Part model, mm, in its own coordinate system. Face numbers are marked on the shaded views. A direction names the side the tool comes from. Round coordinates to 2 decimals unless told otherwise and drop trailing zeros. Write each loop counter-clockwise with the first axis right and the second up, starting at its lowest first coordinate (ties: lowest second). Pieces come first, ordered by that corner, then holes. Notation, with made-up numbers: M 0.25,35.5 L 35.25,35.5 A16 ccw 35.25,55.5 Z; hole C 27,2 d6. An arc over 180 degrees is marked long. Use a Markdown table: item, result. Add a question column.
1) Wall check: probe 1 along Z at (x, y) = (-3, -46); probe 2 along Y at (x, z) = (-14.5, 28); probe 3 along Z at (x, y) = (-27, -83). Give the ranges that are in metal, low to high.
2) Slice it at B-B on x = 1. Write the cut outline in (y, z).
3) Which spindle directions (+Z, -Z, +X, -X, +Y, -Y) get a long thin tool onto all of the face, cutting with end or side? Do the marked faces 1, 2, 3 and 4. Say none if no direction does.
4) Slice it at C-C on z = 51. Write the cut outline in (x, y).
5) Slice it at D-D on y = -47. Write the cut outline in (x, z), plus the area to 3 significant figures.
6) Two-plate mould, pull along Y, no slides. Class the marked faces 5, 6, 7 and 8: released by +Y, released by -Y, zero draft, split by the parting line, or undercut.
7) Drop flat-ended pins along their axis: P1, Ø5, axis at x = 2, y = -102, coming from the +Z side; P2, Ø6, axis at x = -29.5, z = 43.5, coming from the +Y side; P3, Ø12, axis at x = -27.5, z = 90.5, coming from the -Y side. Give the stop position or say it passes through.
8) Slice it at A-A on z = 126.5. Write the cut outline in (x, y).
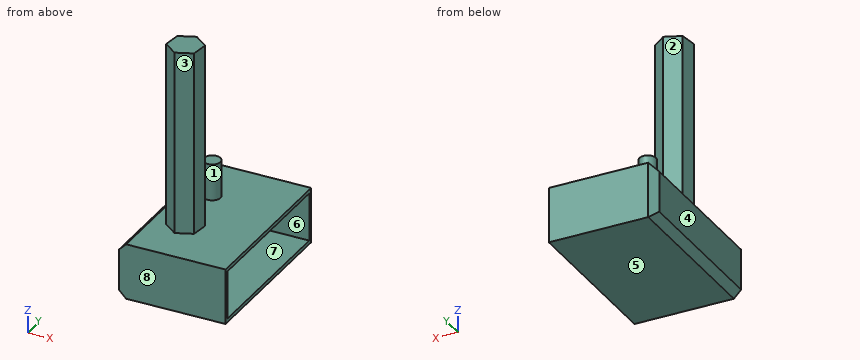
```python
from build123d import *

# Parameters (mm, degrees)
F0_W     = 74.041
F0_H     = 38.5406240821
F1_DEPTH = 115.062
F3_DEPTH = 127.762
F4_R     = 5.7167029037
F5_DEPTH = 25.4
F6_SIZE  = 5.08
F7_SIZE  = 5.08
F8_T     = -2.54


with BuildPart() as f1:
    # F0 (on Front) → F1 (new body)
    with BuildSketch(Plane.XZ):
        with Locations((-20.778500293, 19.270312041)):
            Rectangle(F0_W, F0_H)
    extrude(amount=F1_DEPTH)

    # F2 (on face) → F3 (join)
    with BuildSketch(Plane.XY.offset(38.5406240821)):
        Polygon((-42.2897917902, -81.5107752422), (-32.7059420073, -88.8478676936), (-21.5599086631, -84.2165565412), (-19.9977251018, -72.2481529375), (-29.5815748846, -64.9110604862), (-40.7276082288, -69.5423716385), align=None)
    extrude(amount=F3_DEPTH)

    # F4 (on face) → F5 (join)
    with BuildSketch(Plane.XY.offset(38.5406240821)):
        with Locations((-33.4108434618, -36.7342457175)):
            Circle(F4_R)
    extrude(amount=F5_DEPTH)

    # F6
    f6_edges = [f1.edges().sort_by_distance(p)[0] for p in [
        (-57.799, -57.531, 0),
        (-57.799, 0, 19.270312),
    ]]
    chamfer(f6_edges, length=F6_SIZE)

    # F7
    f7_edges = [f1.edges().sort_by_distance(p)[0] for p in [
        (-57.799, -60.071, 38.540624),
    ]]
    chamfer(f7_edges, length=F7_SIZE)

    # F8
    f8_openings = [f1.faces().sort_by_distance(p)[0] for p in [
        (16.242, -57.531, 19.270312),
    ]]
    offset(amount=F8_T, openings=f8_openings, kind=Kind.INTERSECTION)


solid = f1.part
```
Entries:
| question | item | result |
|---|---|---|
| 1 | probe 1 | z = 0 to 2.54, 36 to 38.54 |
| 1 | probe 2 | y = -115.06 to -112.52, -2.54 to 0 |
| 1 | probe 3 | z = 0 to 2.54, 163.76 to 166.3 |
| 2 | outline | M -115.06,0 L 0,0 L 0,38.54 L -115.06,38.54 Z; hole M -112.52,2.54 L -2.54,2.54 L -2.54,36 L -112.52,36 Z |
| 3 | face 1 | +Z |
| 3 | face 2 | +Z, -X |
| 3 | face 3 | +Z, +X, -Y |
| 3 | face 4 | +Z, -Z, -X, +Y, -Y |
| 4 | outline | M -42.29,-81.51 L -32.71,-88.85 L -21.56,-84.22 L -20,-72.25 L -29.58,-64.91 L -40.73,-69.54 Z; C -33.41,-36.73 d11.43; hole M -39.58,-80.39 L -32.33,-85.94 L -23.89,-82.43 L -22.71,-73.37 L -29.96,-67.82 L -38.4,-71.33 Z; hole C -33.41,-36.73 d6.35 |
| 5 | outline | M -57.8,5.08 L -52.72,0 L 16.24,0 L 16.24,2.54 L -51.67,2.54 L -55.26,6.13 L -55.26,32.41 L -51.67,36 L 16.24,36 L 16.24,38.54 L -52.72,38.54 L -57.8,33.46 Z |
| 5 | area | 448 mm^2 |
| 6 | face 5 | zero draft |
| 6 | face 6 | undercut |
| 6 | face 7 | undercut |
| 6 | face 8 | released by -Y |
| 7 | P1 | stops at z = 38.54 |
| 7 | P2 | stops at y = -31.09 |
| 7 | P3 | stops at y = -88.85 |
| 8 | outline | M -42.29,-81.51 L -32.71,-88.85 L -21.56,-84.22 L -20,-72.25 L -29.58,-64.91 L -40.73,-69.54 Z; hole M -39.58,-80.39 L -32.33,-85.94 L -23.89,-82.43 L -22.71,-73.37 L -29.96,-67.82 L -38.4,-71.33 Z |
